Autodesk Inventor part; units mm, degrees
ref_plane "YZ Plane" through (0, 0, 0) normal (1, 0, 0) x (0, 1, 0)
ref_plane "XZ Plane" through (0, 0, 0) normal (0, 1, 0) x (-1, 0, 0)
ref_plane "XY Plane" through (0, 0, 0) normal (0, 0, 1) x (1, 0, 0)
sketch "Sketch1" plane through (0, 0, 0) normal (0, 1, 0) x (-1, 0, 0)
  line L0 (114.3, 0) -> (114.3, -114.3)
  line L1 (114.3, -114.3) -> (0, -114.3)
  line L2 (25.4, -71.4495) -> (0, -71.4495)
  line L3 (25.4, -46.0495) -> (0, -46.0495)
  line L4 (0, -114.3) -> (0, -71.4495)
  line L5 (114.3, 0) -> (0, 0)
  line L6 (0, 0) -> (0, -46.0495)
  line L7 (25.4, -71.4495) -> (44.45, -71.4495)
  line L8 (44.45, -71.4495) -> (44.45, -46.0495)
  line L9 (44.45, -46.0495) -> (25.4, -46.0495)
extrude "Extrusion1" add sketch "Sketch1" along normal blind 6.35
sketch "Sketch2" plane through (0, 6.35, 0) normal (0, 1, 0) x (1, 0, 0)
  line L0 (-114.3, 0) -> (0, 0)
  line L1 (-114.3, 0) -> (-114.3, 6.35)
  line L2 (-114.3, 114.3) -> (-114.3, 0)
  line L3 (-114.3, 6.35) -> (0, 6.35)
  line L4 (0, 0) -> (0, 46.0495)
  line L5 (0, 0) -> (-114.3, 0)
  line L6 (0, 114.3) -> (-114.3, 114.3)
  line L7 (0, 114.3) -> (0, 107.95)
  line L8 (0, 114.3) -> (0, 71.4495)
  line L9 (0, 107.95) -> (-114.3, 107.95)
  line L10 (-114.3, 114.3) -> (0, 114.3)
extrude "Extrusion2" add sketch "Sketch2" along normal blind 88.9
sketch "Sketch3" plane through (0, 95.25, 0) normal (0, 1, 0) x (1, 0, 0)
  line L0 (-114.3, 6.35) -> (-114.3, 0)
  line L1 (0, 114.3) -> (-114.3, 114.3)
  line L2 (-114.3, 0) -> (0, 0)
  line L3 (0, 0) -> (0, 114.3)
  line L4 (0, 114.3) -> (-114.3, 114.3)
  line L5 (-114.3, 114.3) -> (-114.3, 0)
  point P0 (0, 0)
extrude "Extrusion3" add sketch "Sketch3" along normal blind 6.35
sketch "Sketch4" plane through (0, 6.35, 0) normal (0, 1, 0) x (1, 0, 0)
  line L0 (0, 6.35) -> (0, 46.0495)
  line L1 (0, 107.95) -> (-114.3, 107.95)
  line L2 (0, 6.35) -> (0, 107.95)
  line L3 (0, 6.35) -> (-6.35, 6.35)
  line L4 (-114.3, 6.35) -> (0, 6.35)
  line L5 (-6.35, 6.35) -> (-6.35, 107.95)
  line L6 (0, 71.4495) -> (0, 107.95)
  line L7 (0, 107.95) -> (-6.35, 107.95)
  point P0 (0, 0)
  dimension "d13" = 6.35
extrude "Extrusion4" add sketch "Sketch4" along normal blind 88.9
sketch "Sketch5" plane through (0, 0, 0) normal (1, 0, 0) x (0, 0, -1)
  line L0 (46.0495, 6.35) -> (71.4495, 6.35)
  line L1 (46.0495, 6.35) -> (71.4495, 6.35)
  line L2 (71.4495, 6.35) -> (71.4495, 12.7)
  line L3 (46.0495, 12.7) -> (46.0495, 6.35)
  line L4 (46.0495, 12.7) -> (14.2995, 12.7)
  line L5 (71.4495, 12.7) -> (103.1995, 12.7)
  line L6 (103.1995, 12.7) -> (103.1995, 88.9)
  line L7 (107.95, 95.25) -> (6.35, 95.25)
  line L8 (103.1995, 88.9) -> (14.2995, 88.9)
  line L9 (14.2995, 88.9) -> (14.2995, 12.7)
  point P0 (0, 0)
extrude "Extrusion5" cut sketch "Sketch5" against normal blind 6.35
sketch "Sketch6" plane through (0, 6.35, 0) normal (0, 1, 0) x (1, 0, 0)
  line L0 (-114.3, 107.95) -> (-114.3, 6.35)
  line L1 (-114.3, 6.35) -> (-114.3, 107.95)
  line L2 (-114.3, 107.95) -> (-107.95, 107.95)
  line L3 (-107.95, 107.95) -> (-107.95, 6.35)
  line L4 (-107.95, 6.35) -> (-114.3, 6.35)
  point P0 (0, 0)
extrude "Extrusion6" add sketch "Sketch6" along normal blind 88.9
sketch "Sketch7" plane through (-114.3, 0, -114.3) normal (-1, 0, 0) x (0, 0, 1)
  line L0 (100.0005, 88.9) -> (11.1005, 88.9)
  line L1 (100.0005, 88.9) -> (100.0005, 12.7)
  line L2 (11.1005, 88.9) -> (100.0005, 88.9)
  line L3 (100.0005, 88.9) -> (100.0005, 12.7)
  line L4 (100.0005, 12.7) -> (11.1005, 12.7)
  line L5 (11.1005, 12.7) -> (11.1005, 88.9)
  point P0 (114.3, 0)
extrude "Extrusion7" cut sketch "Sketch7" against normal blind 6.35
sketch "Sketch8" plane through (0, 0, -114.3) normal (0, 0, -1) x (-1, 0, 0)
  line L0 (114.3, 0) -> (0, 0)
  line L1 (6.35, 6.35) -> (107.95, 6.35)
  circle A0 centre (10.8401, 10.8401) radius 4.4901
hole "Hole1" at (-10.8401, 10.8401, -114.3) direction (0, 0, 1) diameter 7.9375 end through all
sketch "Sketch9" plane through (0, 0, -114.3) normal (0, 0, -1) x (-1, 0, 0)
  circle A0 centre (10.8401, 10.8401) radius 3.9687
  circle A1 centre (87.0401, 10.8401) radius 3.9688
  point P0 (0, 0)
hole "Hole2" at (-87.0401, 10.8401, -114.3) direction (0, 0, 1) diameter 7.9375 end through all
sketch "Sketch10" plane through (0, 0, -114.3) normal (0, 0, -1) x (-1, 0, 0)
  circle A0 centre (87.0401, 10.8401) radius 3.9687
  line L0 (87.0401, 10.8401) -> (150.5401, 10.8401) construction
  circle A1 centre (76.0135, 73.3754) radius 14
  point P0 (0, 0)
hole "Hole3" at (-76.0135, 73.3754, -114.3) direction (0, 0, 1) diameter 28 end through all
sketch "Sketch11" plane through (0, 101.6, 0) normal (0, 1, 0) x (1, 0, 0)
  point P0 (0, 0)
properties part number "Chasis_rework"
CAD build for the part. Positions are in the model's coordinates, mm. A direction names the side the tool comes from. Round coordinates to 2 decimals unless told otherwise and drop trailing zeros. Order: outer loops, then holes, each group sorted by start corner. A loop starts at its lowest first (then second) coordinate and runs counter-clockwise, first axis right, second up. Notation, with made-up numbers: (76, 63) - (91, 63) arc R28 cw to (91, 83) - close; hole circle Ø3 at (2, 37.25). An arc over 180 degrees is marked (long way). Return JSON: item names as keys, results as strings.
(1) Cut at B-B (z = -58). Give the cut face in (x, y), then the cut area to 3 significant figures.
Answer key:
{"outline": "(-114.3, 0) - (-44.45, 0) - (-44.45, 6.35) - (-107.95, 6.35) - (-107.95, 12.7) - (-114.3, 12.7) - close; (-114.3, 88.9) - (-107.95, 88.9) - (-107.95, 95.25) - (-6.35, 95.25) - (-6.35, 88.9) - (0, 88.9) - (0, 101.6) - (-114.3, 101.6) - close", "area": "1,290 mm^2"}
(2) Pull direction X, two halves, no side cores. Call faces 1 (the face through (-3, 12.7, -30)), 2 (the face through (-114.3, 95, -58)), 3 (the face through (-90.975, 10.323, -111.081)), 4 (the face through (-44.45, 3, -59)): +X half, -X half, draft (parallel to the pull), parting line (faces both ways), or undercut.
Answer key:
{"face 1": "draft", "face 2": "-X half", "face 3": "undercut", "face 4": "+X half"}
(3) Wall check: probe 1 along Z at (x, y) = (-32, 73); probe 2 along Y at (x, z) = (-69, -56). Give the ranges that are in metal, low to high. Write a range as from..to.
Answer key:
{"probe 1": "z = -114.3..-107.95, -6.35..0", "probe 2": "y = 0..6.35, 95.25..101.6"}
(4) Tool access for faces 5 (the face through (-111, 50, -103.2)), 6 (the face through (-90.975, 10.323, -3.131)), 7 (the face through (-107.95, 90, -46)): list every direction of +Z, -Z, +X, -X, +Y, -Y with a clear straight run to the whole face (end or side of a thin tool).
Answer key:
{"face 5": "+X, -X", "face 6": "+Z, -Z", "face 7": "none"}
(5) Cut at D-D (x = -79.5). Give the cut face in (y, z), then the cut area to 3 significant figures.
Answer key:
{"outline": "(0, -114.3) - (59.82, -114.3) - (59.82, -107.95) - (6.35, -107.95) - (6.35, -6.35) - (59.82, -6.35) - (59.82, 0) - (0, 0) - close; (86.93, -114.3) - (101.6, -114.3) - (101.6, 0) - (86.93, 0) - (86.93, -6.35) - (95.25, -6.35) - (95.25, -107.95) - (86.93, -107.95) - close", "area": "2,240 mm^2"}
(6) Cut at A-A (y = 28). Give the cut face in (x, z), then the cut area to 3 significant figures.
Answer key:
{"outline": "(-114.3, -114.3) - (0, -114.3) - (0, -103.2) - (-6.35, -103.2) - (-6.35, -107.95) - (-107.95, -107.95) - (-107.95, -103.2) - (-114.3, -103.2) - close; (-114.3, -14.3) - (-107.95, -14.3) - (-107.95, -6.35) - (-6.35, -6.35) - (-6.35, -14.3) - (0, -14.3) - (0, 0) - (-114.3, 0) - close", "area": "1,610 mm^2"}
(7) Pin check, flat tips, straight feed: pin 1 Ø2 at (x, z) = (-37.5, -60) entering from -Y; pin 2 Ø2 at (x, y) = (-99, 42) entering from +Z; pin 3 Ø3 at (y, z) = (3, -62) entering from +X; pin 4 Ø3 at (x, z) = (-2, -55) entering from -Y. Stop position of each tip, or through.
Answer key:
{"pin 1": "stops at y = 95.25", "pin 2": "stops at z = 0", "pin 3": "stops at x = -44.45", "pin 4": "stops at y = 88.9"}
(8) Cut at C-C (y = 91). Give the cut face in (x, z), then the cut area to 3 significant figures.
Answer key:
{"outline": "(-114.3, -114.3) - (0, -114.3) - (0, 0) - (-114.3, 0) - close; hole (-107.95, -107.95) - (-6.35, -107.95) - (-6.35, -6.35) - (-107.95, -6.35) - close", "area": "2,740 mm^2"}
